Here's how the part is built. I have some questions about the finished solid (model axes, mm). Face numbers are marked on the shaded views. A direction names the side the tool comes from. Give positions to 0.01 mm unless a question says otherwise; leave off trailing zeros. Loops run counter-clockwise (first coordinate to the right, second up) from the corner with the lowest first, then second, coordinate; pieces in that order, holes last. Notation, with made-up numbers: (40, -17.5) - (66, -17.5) arc R29 cw to (66, 7.5) - close; hole circle Ø7 at (12, -27.75). An arc over 180 degrees is marked (long way). Return JSON: item names as keys, results as strings. Group by question number.
(1) For P1, Ø3, axis at x = -2, z = -3.5, coming from the +Y side; P2, Ø0.8, axis at y = 2, z = -1.5, coming from the +X side; P3, Ø1.7, axis at x = 1.5, y = 1, coming from the +Z side; P4, Ø1.5, axis at x = 0, z = -0.5, coming from the +Y side, each with a flat end and sliding along its axis, tell me the tip position at first contact or that it passes through.
(2) If we section it at A-A (z = 0): Please give me the cut outline in (x, y), then the cut area to 3 significant figures.
(3) If we mould it in two halves opening along X, with no side actions, what happens to the marked faces 1, 2 and 3? For each: released by +X, released by -X, zero draft, split by the parting line, or undercut.
(4) If we section it at D-D (x = 4.25): Please give me the cut outline in (y, z).
(5) On a 3-axis mill with a long thin cutter (end or side, diameter ignored), from which of +Z, -Z, +X, -X, +Y, -Y can I reach the whole of each face in a straight line? I mean the marked faces 4 and 5. Say none if no direction works.
(6) If we section it at B-B (x = 0): Please give me the cut outline in (y, z).
(7) If we section it at C-C (y = 5.5): Please give me the cut outline in (x, z).
(8) I need wall thicknesses on probe 1 along Y at (x, z) = (-3, -1.5); probe 2 along X at (y, z) = (0.75, 0.5); probe 3 along Z at (x, y) = (4.25, 3.5). Which ranges of each line are inside material? Lowest first, please. Write a range as [from, to].
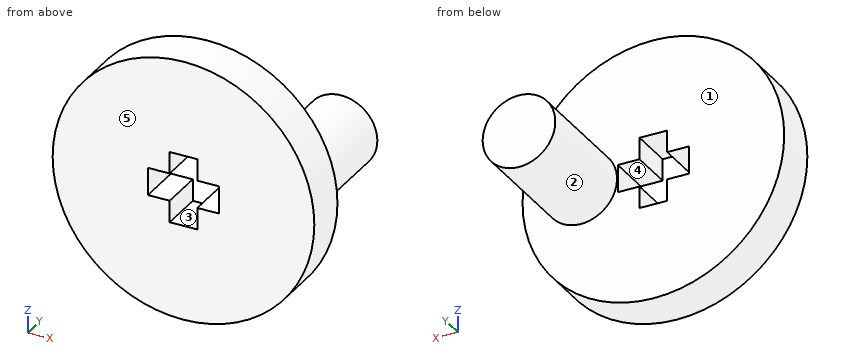
```python
from build123d import *

# Parameters (mm, degrees)
SKETCH1_R           = 9
BOSS_EXTRUDE1_DEPTH = 3
SKETCH2_R           = 2.5
BOSS_EXTRUDE2_DEPTH = 8


with BuildPart() as part:
    # Sketch1 → Boss-Extrude1 (new body)
    with BuildSketch(Plane(origin=(0, 0, 0), x_dir=(1, 0, 0), z_dir=(0, 1, 0))):
        Circle(SKETCH1_R)
        Polygon((-2.45, 0.95), (-2.45, -0.95), (-0.95, -0.95), (-0.95, -2.45), (0.95, -2.45), (0.95, -0.95), (2.45, -0.95), (2.45, 0.95), (0.95, 0.95), (0.95, 2.45), (-0.95, 2.45), (-0.95, 0.95), align=None, mode=Mode.SUBTRACT)
    extrude(amount=BOSS_EXTRUDE1_DEPTH)

    # Sketch2 → Boss-Extrude2 (add)
    with BuildSketch(Plane(origin=(0, 3, 0), x_dir=(1, 0, 0), z_dir=(0, 1, 0))):
        with Locations((5, 0)):
            Circle(SKETCH2_R)
    extrude(amount=BOSS_EXTRUDE2_DEPTH)


solid = part.part
```
Values:
{
 "1": {"P1": "y = 3", "P2": "x = 8.93", "P3": "z = 8.98", "P4": "through"},
 "2": {"outline": "(-9, 0) - (-2.45, 0) - (-2.45, 3) - (-9, 3) - close; (2.45, 0) - (9, 0) - (9, 3) - (7.5, 3) - (7.5, 11) - (2.5, 11) - (2.5, 3) - (2.45, 3) - close", "area": "79.3 mm2"},
 "3": {"face 1": "zero draft", "face 2": "split by the parting line", "face 3": "undercut"},
 "4": {"outline": "(0, -7.93) - (3, -7.93) - (3, -2.38) - (11, -2.38) - (11, 2.38) - (3, 2.38) - (3, 7.93) - (0, 7.93) - close"},
 "5": {"face 4": "+Y, -Y", "face 5": "+Z, -Z, +X, -X, -Y"},
 "6": {"outline": "(0, -9) - (3, -9) - (3, -2.45) - (0, -2.45) - close; (0, 2.45) - (3, 2.45) - (3, 9) - (0, 9) - close"},
 "7": {"outline": "circle Ø5 at (5, 0)"},
 "8": {"probe 1": "[0, 3]", "probe 2": "[-8.99, -2.45], [2.45, 8.99]", "probe 3": "[-2.38, 2.38]"}
}
